from build123d import *

# Parameters (mm, degrees)
SKETCH_1_R          = 75
SKETCH_1_R_2        = 1.5
SKETCH_1_R_3        = 20
EXTRUDE_1_DEPTH     = 7
SKETCH_2_R          = 2.5
CUT_EXTRUDE_1_DEPTH = 4
EXTRUDE_2_DEPTH     = 7
EXTRUDE_3_DEPTH     = 7
EXTRUDE_4_DEPTH     = 7
SKETCH_6_W          = 6.673333333
SKETCH_6_H          = 7
CUT_EXTRUDE_2_DEPTH = 7


with BuildPart() as part:
    # 草图1 → 凸台-拉伸1 (new body)
    with BuildSketch(Plane.XY):
        with Locations(Location((0, 0, 0), (0, 0, 180))):
            Circle(SKETCH_1_R)
        with BuildLine():
            ThreePointArc((-3.219389508, -67.923747918), (-48.083261121, -48.083261121), (-67.923747918, -3.219389508))
            Line((-67.923747918, -3.219389508), (-59, -3.219389508))
            Line((-59, -3.219389508), (-39.870233649, -3.219389508))
            ThreePointArc((-39.870233649, -3.219389508), (-28.284271247, -28.284271247), (-3.219389508, -39.870233649))
            Line((-3.219389508, -39.870233649), (-3.219389508, -67.923747918))
        make_face(mode=Mode.SUBTRACT)
        with Locations(Location((0, -27.5, 0), (0, 0, 180))):
            Circle(SKETCH_1_R_2, mode=Mode.SUBTRACT)
        with BuildLine():
            Line((39.870233649, -3.219389508), (67.923747918, -3.219389508))
            ThreePointArc((67.923747918, -3.219389508), (48.083261121, -48.083261121), (3.219389508, -67.923747918))
            Line((3.219389508, -67.923747918), (3.219389508, -59))
            Line((3.219389508, -59), (3.219389508, -39.870233649))
            ThreePointArc((3.219389508, -39.870233649), (28.284271247, -28.284271247), (39.870233649, -3.219389508))
        make_face(mode=Mode.SUBTRACT)
        with Locations(Location((27.5, 0, 0), (0, 0, 180))):
            Circle(SKETCH_1_R_2, mode=Mode.SUBTRACT)
        with Locations(Location((-27.5, 0, 0), (0, 0, 180))):
            Circle(SKETCH_1_R_2, mode=Mode.SUBTRACT)
        with BuildLine():
            ThreePointArc((-67.923747918, 3.219389508), (-48.083261121, 48.083261121), (-3.219389508, 67.923747918))
            Line((-3.219389508, 67.923747918), (-3.219389508, 59))
            Line((-3.219389508, 59), (-3.219389508, 39.870233649))
            ThreePointArc((-3.219389508, 39.870233649), (-28.284271247, 28.284271247), (-39.870233649, 3.219389508))
            Line((-39.870233649, 3.219389508), (-59.015976915, 3.219389508))
            Line((-59.015976915, 3.219389508), (-67.923747918, 3.219389508))
        make_face(mode=Mode.SUBTRACT)
        with Locations(Location((0, 0, 0), (0, 0, 180))):
            Circle(SKETCH_1_R_3, mode=Mode.SUBTRACT)
        with Locations(Location((0, 27.5, 0), (0, 0, 180))):
            Circle(SKETCH_1_R_2, mode=Mode.SUBTRACT)
        with BuildLine():
            Line((3.219389508, 39.870233649), (3.219389508, 67.923747918))
            ThreePointArc((3.219389508, 67.923747918), (48.083261121, 48.083261121), (67.923747918, 3.219389508))
            Line((67.923747918, 3.219389508), (59, 3.219389508))
            Line((59, 3.219389508), (39.870233649, 3.219389508))
            ThreePointArc((39.870233649, 3.219389508), (28.284271247, 28.284271247), (3.219389508, 39.870233649))
        make_face(mode=Mode.SUBTRACT)
    extrude(amount=EXTRUDE_1_DEPTH)

    # 草图2 → 切除-拉伸1 (cut)
    with BuildSketch(Plane.XY):
        with Locations((27.5, 0)):
            Circle(SKETCH_2_R)
        with Locations((0, -27.5)):
            Circle(SKETCH_2_R)
        with Locations((-27.5, 0)):
            Circle(SKETCH_2_R)
        with Locations((0, 27.5)):
            Circle(SKETCH_2_R)
    extrude(amount=CUT_EXTRUDE_1_DEPTH, mode=Mode.SUBTRACT)

    # 草图3 → 凸台-拉伸2 (add)
    with BuildSketch(Plane(origin=(0, -75, 0), x_dir=(1, 0, 0), z_dir=(0, 1, 0))):
        Polygon((-75, 0), (-75, -3.5), (-75, -78.5), (0, -14), (75, -78.5), (75, 0), (0, 0), align=None)
    extrude(amount=EXTRUDE_2_DEPTH)

    # 草图4 → 凸台-拉伸3 (add)
    with BuildSketch(Plane.XY):
        with BuildLine():
            Line((-75, 0), (-75, -75))
            Line((-75, -75), (75, -75))
            Line((75, -75), (75, 0))
            Line((75, 0), (68, 0))
            ThreePointArc((68, 0), (0, -68), (-68, 0))
            Line((-68, 0), (-75, 0))
        make_face()
    extrude(amount=EXTRUDE_3_DEPTH)

    # 草图5 → 凸台-拉伸4 (add)
    with BuildSketch(Plane(origin=(-75, 0, 0), x_dir=(0, 0, -1), z_dir=(1, 0, 0))):
        Polygon((0, 0), (-7, 0), (-78.5, -75), (0, -75), align=None)
    extrude_4 = extrude(amount=EXTRUDE_4_DEPTH)

    # 镜向1: 凸台-拉伸4 across plane
    add(extrude_4.mirror(Plane(origin=(0, 0, 0), x_dir=(0, 0, 1), z_dir=(1, 0, 0))))

    # 草图6 → 切除-拉伸2 (cut)
    with BuildSketch(Plane(origin=(-75, 0, 0), x_dir=(0, 0, -1), z_dir=(1, 0, 0))):
        with Locations((-75.163333333, -71.5)):
            Rectangle(SKETCH_6_W, SKETCH_6_H)
    cut_extrude_2 = extrude(amount=CUT_EXTRUDE_2_DEPTH, mode=Mode.SUBTRACT)

    # 镜向5: 切除-拉伸2 across plane
    add(cut_extrude_2.mirror(Plane(origin=(0, 0, 0), x_dir=(0, 0, 1), z_dir=(1, 0, 0))), mode=Mode.SUBTRACT)


solid = part.part
Geometry check sheet. Reference: the model listing, model coordinates, mm. A direction names the side the tool comes from. Round coordinates to 2 decimals unless told otherwise and drop trailing zeros. Loops run counter-clockwise (first coordinate to the right, second up) from the corner with the lowest first, then second, coordinate; pieces in that order, holes last.
Item 1: Cross-section at B-B on x = -57.5. Record the boundary of the cut face in (y, z), then the cut area to 3 significant figures.
Item 2: Cross-section at A-A on y = 56.5. Record the boundary of the cut face in (x, z), then the cut area to 3 significant figures.
Item 3: Mould release check, pull along Y, two halves, no side actions. Record for faces 1 (the flat face through (33.524, -71.549, 42.831)), 2 (the cylindrical face through (-28.562, -28.004, 3.451)), 3 (the flat face through (71.549, -33.524, 38.96)), 4 (the flat face through (-1, -75, 12)): pulls with the +Y half, pulls with the -Y half, needs draft (parallel to the pull), parting line crosses it, or undercut.
Item 4: Access from +Z, -Z, +X, -X, +Y, -Y to the whole of each face (thin tool, end or side, straight path). Record for faces 5 (the flat face through (-68, -49, 25)), 6 (the cylindrical face through (-47.58, -48.58, 3.45)), 7 (the flat face through (-26, -1, 4)).
Item 5: Gauge pin test, flat ends, axial feed: pin 1 (2 mm diameter, centred on x = 73, y = -70, fed in from +Z); pin 2 (5.5 mm diameter, centred on y = 59, z = 5, fed in from -X); pin 3 (4 mm diameter, centred on x = 45.5, z = 37, fed in from +Y); pin 4 (2.5 mm diameter, centred on x = 27.5, y = 0, fed in from -Z). Record the tip position at first contact, or that the pin passes through.
Item 6: Cross-section at C-C on z = 49. Record the boundary of the cut face in (x, y), then the cut area to 3 significant figures.
Item 7: Cross-section at D-D on y = -34. Record the boundary of the cut face in (x, z), then the cut area to 3 significant figures.
Item 8: Thickness scan on line 1 (Y direction, x = 0, z = 1.75); line 2 (Y direction, x = 0, z = 5); line 3 (X direction, y = -50, z = 8). Record the ranges inside material, lowest first.
Answer sheet:
1. outline: (-75, 0) - (-36.3, 0) - (-36.3, 7) - (-68, 7) - (-68, 63.45) - (-75, 63.45) - close; (-3.22, 0) - (3.22, 0) - (3.22, 7) - (-3.22, 7) - close; (36.3, 0) - (48.15, 0) - (48.15, 7) - (36.3, 7) - close
1. area: 794 mm2
2. outline: (-49.32, 0) - (-37.84, 0) - (-37.84, 7) - (-49.32, 7) - close; (-3.22, 0) - (3.22, 0) - (3.22, 7) - (-3.22, 7) - close; (37.84, 0) - (49.32, 0) - (49.32, 7) - (37.84, 7) - close
2. area: 206 mm2
3. face 1: needs draft
3. face 2: undercut
3. face 3: pulls with the +Y half
3. face 4: pulls with the -Y half
4. face 5: +Z, +Y
4. face 6: +Z, -Z
4. face 7: -Z
5. pin 1: stops at z = 71.83
5. pin 2: stops at x = -49.61
5. pin 3: stops at y = -68
5. pin 4: passes through
6. outline: (-75, -75) - (-40.7, -75) - (-40.7, -68) - (-68, -68) - (-68, -44.06) - (-75, -44.06) - close; (40.7, -75) - (75, -75) - (75, -44.06) - (68, -44.06) - (68, -68) - (40.7, -68) - close
6. area: 815 mm2
7. outline: (-75, 0) - (-58.89, 0) - (-58.89, 7) - (-68, 7) - (-68, 39.41) - (-75, 39.41) - close; (-21.07, 0) - (21.07, 0) - (21.07, 7) - (-21.07, 7) - close; (58.89, 0) - (75, 0) - (75, 39.41) - (68, 39.41) - (68, 7) - (58.89, 7) - close
7. area: 974 mm2
8. line 1: y = -75 to -30, -25 to -20, 20 to 25, 30 to 75
8. line 2: y = -75 to -29, -26 to -20, 20 to 26, 29 to 75
8. line 3: x = -75 to -68, 68 to 75
